Design review of the part built by this model. Coordinates are the model's own, in mm. Face numbers are marked on the shaded views. A direction names the side the tool comes from. Coordinates: 2 decimals unless noted, no trailing zeros. Loops run counter-clockwise (first coordinate to the right, second up) from the corner with the lowest first, then second, coordinate; pieces in that order, holes last. Notation, with made-up numbers: (-8.75, -4.75) -> (42.25, -4.75) arc R26 ccw to (42.25, 18.25) -> close; hole circle Ø8 at (83.5, 38). An arc over 180 degrees is marked (long way). Answer in a Markdown table with one row per item.
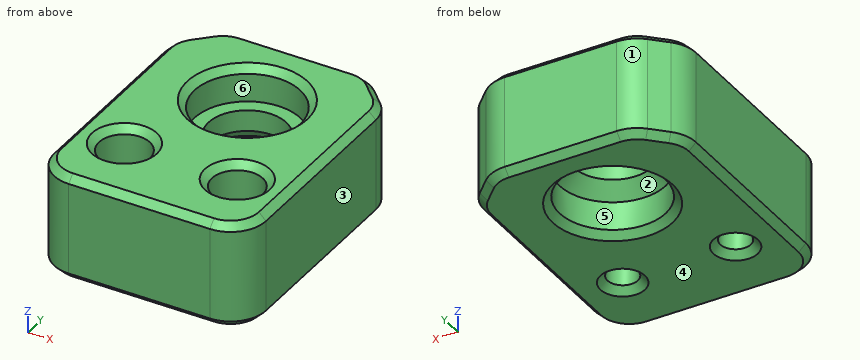
```python
from build123d import *

# Parameters (mm, degrees)
F0_W     = 30
F0_H     = 38.5
F0_R     = 3.6
F0_R_2   = 7.5
F1_DEPTH = 15
F0_R_3   = 2.15
F2_DEPTH = 5
F3_START = 5
F0_R_4   = 5.5
F3_DEPTH = 5
F4_SIZE  = 1.99999
F5_SIZE  = 5
F6_R     = 5
F7_R     = 5
F8_SIZE  = 1


# Not quite as in the source:
# - a fillet or chamfer is up to 0.001 mm smaller than in the source, because OpenCascade refuses the exact size


with BuildPart() as f1:
    # F0 (on Top) → F1 (new body)
    with BuildSketch(Plane.XY):
        Rectangle(F0_W, F0_H)
        with Locations((-8, -9.25)):
            Circle(F0_R, mode=Mode.SUBTRACT)
        with Locations((8, -9.25)):
            Circle(F0_R, mode=Mode.SUBTRACT)
        with Locations((0, 6.75)):
            Circle(F0_R_2, mode=Mode.SUBTRACT)
    extrude(amount=F1_DEPTH)

    # F0 (on Top) → F2 (join)
    with BuildSketch(Plane.XY):
        with Locations((-8, -9.25)):
            Circle(F0_R)
        with Locations((-8, -9.25)):
            Circle(F0_R_3, mode=Mode.SUBTRACT)
        with Locations((8, -9.25)):
            Circle(F0_R)
        with Locations((8, -9.25)):
            Circle(F0_R_3, mode=Mode.SUBTRACT)
    extrude(amount=F2_DEPTH)

    # F0 (on Top) → F3 (join)
    with BuildSketch(Plane.XY.offset(F3_START)):
        with Locations((0, 6.75)):
            Circle(F0_R_2)
        with Locations((0, 6.75)):
            Circle(F0_R_4, mode=Mode.SUBTRACT)
    extrude(amount=F3_DEPTH)

    # F4 (size 2 in the source; OpenCascade refuses exactly that, so slightly less here)
    f4_edges = [f1.edges().sort_by_distance(p)[0] for p in [
        (-5.5, 6.75, 5),
    ]]
    chamfer(f4_edges, length=F4_SIZE)

    # F5
    f5_edges = [f1.edges().sort_by_distance(p)[0] for p in [
        (15, 19.25, 7.5),
        (-15, 19.25, 7.5),
    ]]
    chamfer(f5_edges, length=F5_SIZE)

    # F6
    f6_edges = [f1.edges().sort_by_distance(p)[0] for p in [
        (15, -19.25, 7.5),
        (-15, -19.25, 7.5),
    ]]
    fillet(f6_edges, radius=F6_R)

    # F7
    f7_edges = [f1.edges().sort_by_distance(p)[0] for p in [
        (15, 14.25, 7.5),
        (10, 19.25, 7.5),
        (-10, 19.25, 7.5),
        (-15, 14.25, 7.5),
    ]]
    fillet(f7_edges, radius=F7_R)

    # F8
    f8_edges = [f1.edges().sort_by_distance(p)[0] for p in [
        (15, -1.035534, 15),
        (14.619398, 14.092349, 15),
        (13.535534, -17.785534, 15),
        (12.5, 16.75, 15),
        (0, -19.25, 15),
        (9.842349, 18.869398, 15),
        (-13.535534, -17.785534, 15),
        (0, 19.25, 15),
        (-15, -1.035534, 15),
        (-9.842349, 18.869398, 15),
        (-14.619398, 14.092349, 15),
        (-12.5, 16.75, 15),
        (-11.6, -9.25, 15),
        (4.4, -9.25, 15),
        (-7.5, 6.75, 15),
        (15, -1.035534, 0),
        (14.619398, 14.092349, 0),
        (13.535534, -17.785534, 0),
        (12.5, 16.75, 0),
        (0, -19.25, 0),
        (9.842349, 18.869398, 0),
        (-13.535534, -17.785534, 0),
        (0, 19.25, 0),
        (-15, -1.035534, 0),
        (-9.842349, 18.869398, 0),
        (-14.619398, 14.092349, 0),
        (-12.5, 16.75, 0),
        (-7.5, 6.75, 0),
        (-10.15, -9.25, 0),
        (5.85, -9.25, 0),
    ]]
    chamfer(f8_edges, length=F8_SIZE)


solid = f1.part
```
(1) For pin 1 (17.5 mm diameter, centred on x = 0, y = 6.75, fed in from -Z); pin 2 (5.5 mm diameter, centred on x = 8, y = -9.25, fed in from -Z); pin 3 (3.5 mm diameter, centred on x = -8, y = -9.25, fed in from +Z); pin 4 (8.5 mm diameter, centred on x = 8, y = -9.25, fed in from +Z), all flat-tipped, find the tip position at first contact; note any pin that passes through.
Evaluation:
| item | result |
|---|---|
| pin 1 | stops at z = 0 |
| pin 2 | stops at z = 0.4 |
| pin 3 | passes through |
| pin 4 | stops at z = 14.65 |
(2) Take a section at D-D on z = 7.5. Give the boundary of the cut face in (x, y).
Evaluation:
| item | result |
|---|---|
| outline | (-15, -14.25) arc R5 ccw to (-10, -19.25) -> (10, -19.25) arc R5 ccw to (15, -14.25) -> (15, 12.18) arc R5 ccw to (13.54, 15.71) -> (11.46, 17.79) arc R5 ccw to (7.93, 19.25) -> (-7.93, 19.25) arc R5 ccw to (-11.46, 17.79) -> (-13.54, 15.71) arc R5 ccw to (-15, 12.18) -> close; hole circle Ø7.2 at (-8, -9.25); hole circle Ø11 at (0, 6.75); hole circle Ø7.2 at (8, -9.25) |
(3) Draft analysis for pull direction X (two halves, no side actions). For the marked faces 1, 2 and 3, state which applies: pulls with the +X half, pulls with the -X half, needs draft (parallel to the pull), parting line crosses it, or undercut.
Evaluation:
| item | result |
|---|---|
| face 1 | pulls with the -X half |
| face 2 | undercut |
| face 3 | pulls with the +X half |
(4) To check wall thickness, follow probe 1 along Y at (x, z) = (7.75, 13); probe 2 along Y at (x, z) = (0, 9); probe 3 along X at (y, z) = (2, 12). State the ranges of each line that lie inside material, in increasing order.
Evaluation:
| item | result |
|---|---|
| probe 1 | y = -19.25 to -12.84, -5.66 to 19.25 |
| probe 2 | y = -19.25 to 1.25, 12.25 to 19.25 |
| probe 3 | x = -15 to -5.8, 5.8 to 15 |
(5) Tool access review of the marked faces 4, 5 and 6: name each direction out of +Z, -Z, +X, -X, +Y, -Y from which nothing blocks a thin tool from reaching the whole face with its end or side.
Evaluation:
| item | result |
|---|---|
| face 4 | -Z, +X, -X, +Y, -Y |
| face 5 | -Z |
| face 6 | +Z |
(6) Take a section at A-A on y = -9.25. Count the separate pieces of the cut face and the enclosed holes in it, and give its area (3 significant figures).
Evaluation:
| item | result |
|---|---|
| separate pieces | 3 |
| enclosed holes | 0 |
| area | 257 mm² |
